from build123d import *

# Parameters (mm, degrees)
F0_W     = 38.1
F0_H     = 590.55
F1_DEPTH = 19.05
F3_DEPTH = 38.1
F5_DEPTH = 38.101


with BuildPart() as f1:
    # F0 (on Front) → F1 (new body, symmetric)
    with BuildSketch(Plane.XZ):
        Rectangle(F0_W, F0_H)
    extrude(amount=F1_DEPTH, both=True)

    # F2 (on face) → F3 (cut, through all)
    with BuildSketch(Plane.XZ.offset(19.05)):
        Polygon((19.05, 168.275), (6.35, -295.275), (19.05, -295.275), align=None)
    extrude(amount=-F3_DEPTH, mode=Mode.SUBTRACT)

    # F4 (on face) → F5 (cut, through all)
    with BuildSketch(Plane.YZ.offset(19.05)):
        Polygon((19.05, -295.275), (19.05, 168.275), (6.35, -295.275), align=None)
    extrude(amount=-F5_DEPTH, mode=Mode.SUBTRACT)


solid = f1.part
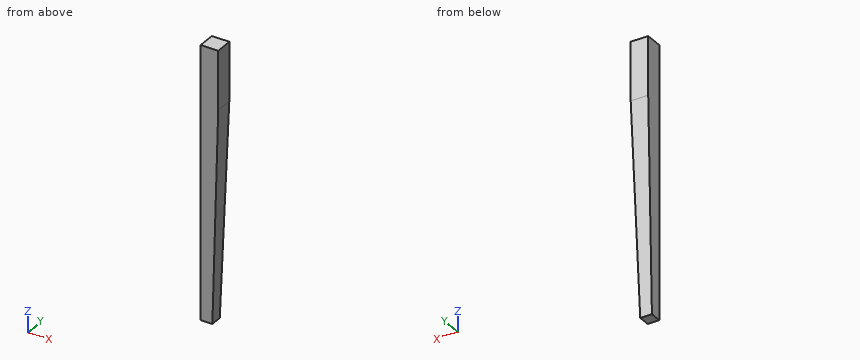
The listing builds one solid part. Answer for the finished solid, in the listing's coordinates (mm). Coordinates: 2 decimals unless noted, no trailing zeros. Loops run counter-clockwise (first coordinate to the right, second up) from the corner with the lowest first, then second, coordinate; pieces in that order, holes last. Notation, with made-up numbers: (2, 74.5) -> (56, 74.5) arc R6 cw to (56, 83.5) -> close; hole circle Ø8 at (-29, 76.25). An arc over 180 degrees is marked (long way). Answer in a Markdown table with one row per item. Add a question column.
1. The part is cut by section A-A, the plane x = -9.5. Write down the section's boundary in (y, z) (3 decimals), then the cut area to 3 significant figures.
2. The part is cut by section C-C, the plane z = 156. Write down the section's boundary in (x, y).
3. Consider line 1 (Y direction, x = 7.5, z = -98); line 2 (Y direction, x = -6, z = -150.5); line 3 (X direction, y = -9, z = -134). Determine where each line is inside the solid, lowest interval first. Write a range as [from, to].
4. Flat-ended cylindrical pins translate along their axes: P1, Ø3, axis at x = 5.5, z = -203, coming from the +Y side; P2, Ø4, axis at y = -11.5, z = 131, coming from the +X side; P3, Ø1.5, axis at x = -2, z = 55.5, coming from the +Y side. Find the tip coordinate at first contact, or state that the pin passes through.
5. The part is cut by section D-D, the plane z = -98.5. Write down the section's boundary in (x, y), then the cut area to 3 significant figures.
Answer below:
| question | item | result |
|---|---|---|
| 1 | outline | (-19.05, -295.275) -> (6.35, -295.275) -> (19.05, 168.275) -> (19.05, 295.275) -> (-19.05, 295.275) -> close |
| 1 | area | 19,600 mm2 |
| 2 | outline | (-19.05, -19.05) -> (18.71, -19.05) -> (18.71, 18.71) -> (-19.05, 18.71) -> close |
| 3 | line 1 | [-19.05, 11.75] |
| 3 | line 2 | [-19.05, 10.32] |
| 3 | line 3 | [-19.05, 10.77] |
| 4 | P1 | y = 8.92 |
| 4 | P2 | x = 18.08 |
| 4 | P3 | y = 15.98 |
| 5 | outline | (-19.05, -19.05) -> (11.74, -19.05) -> (11.74, 11.74) -> (-19.05, 11.74) -> close |
| 5 | area | 948 mm2 |
